Autodesk Inventor part; units mm, degrees
ref_plane "IDS_WORKPLANE{1}" through (-0.8, 0, 0) normal (1, 0, 0) x (0, 1, 0)
ref_plane "Work Plane2" through (3.5, 0, 0) normal (0, 0, -1) x (1, 0, 0)
ref_plane "YZ Plane" through (0, 0, 0) normal (1, 0, 0) x (0, 1, 0)
sketch "Sketch1" plane through (0, 0, 0) normal (0, 0, 1) x (1, 0, 0)
  line L0 (13, 0) -> (13, 1.75)
  line L1 (13, 1.75) -> (2.35, 1.75)
  line L2 (0.45, 3.65) -> (0, 3.65)
  line L3 (0, 3.65) -> (0, 0) construction
  arc A0 (0, 3.65) -> (-0.8, 0) centre (7.9266, 0) ccw
  line L4 (-3.7972, 0) -> (15.7995, 0)
  line L5 (0, -0.7387) -> (0, 4.432)
  line L6 (-0.8, 0) -> (-0.8, 3.65) construction
  line L7 (-0.8, 3.65) -> (0, 3.65) construction
  line L8 (0, 3.65) -> (0, 0)
  line L9 (-0.8, 0) -> (0, 0)
  line L10 (0, 0) -> (13, 0)
  line L11 (0.45, 3.65) -> (2.35, 1.75)
  dimension "d0" = 0.8
  dimension "d1" = 3.5
  dimension "d2" = 7.3
  dimension "d11" = 45
  dimension "d14" = 2.35
  dimension "d15" = 10.65
revolve "Body" add sketch "Sketch1" angle 360 about axis through (0, 0, 0) along (1, 0, 0)
ref_plane "IDS_WORKPLANE{1}" through (-0.8, 0, 0) normal (1, 0, 0) x (0, 1, 0)
sketch "Sketch2" plane through (-0.8, 0, 0) normal (1, 0, 0) x (0, 1, 0)
  line L0 (0, -5.11) -> (0, 5.11)
  line L1 (-5.11, 0) -> (5.11, 0)
  line L2 (0.5, -3.65) -> (-0.5, -3.65)
  line L3 (-0.5, -3.65) -> (-0.5, 3.65)
  line L4 (-0.5, 3.65) -> (0.5, 3.65)
  line L5 (0.5, 3.65) -> (0.5, -3.65)
  line L6 (0, 3.65) -> (0, -3.65) construction
  line L7 (-0.5, 0) -> (0.5, 0) construction
  circle A0 centre (0, 0) radius 3.65
  dimension "d8" = 1
extrude "Slot" cut sketch "Sketch2" along normal blind 1.4 contours A0 L3 L1 L0 | A0 L5 L2 | L2 L3 A0 | L0 L1 L5 A0 | L1 L3 A0 L0 | L0 A0 L5 L1 | A0 L3 L4 | L4 L5 A0
thread "Thread"
chamfer "Chamfer1" distance 1.75 distance2 3.2 1 edges at (13, -1.75, 0) measured on face at (13, -0.4366, 0.1076)
ref_plane "Work Plane2" through (3.5, 0, 0) normal (0, 0, -1) x (1, 0, 0)
equation "\"d0\" = KR"
equation "\"d1\" = NND"
equation "\"d2\" = KOD"
equation "\"d11\" = 0.5 * SEWI"
equation "\"d14\" = KOH"
equation "\"d15\" = GEL"
equation "\"d8\" = SBR"
equation "\"d9\" = STI"
equation "\"d3\" = GEL"
equation "\"d5\" = -0.5 * GD2 + 0.5 * NND"
equation "\"d6\" = SPTZ"
equation "\"NND\" = 3.5"
equation "\"GEL\" = 10.65"
equation "\"KOD\" = 7.3"
equation "\"KOH\" = 2.35"
equation "\"STI\" = 1.4"
equation "\"SBR\" = 1"
equation "\"KR\" = 0.8"
equation "\"SPTZ\" = 3.2"
equation "\"GD2\" = 0"
equation "\"SEWI\" = 90deg"
equation "\"d7\" = -KR"
equation "\"EPV\" = 4.1"
equation "\"THREADDIA\" = 3.5"
equation "\"TOA\" = 30deg"
equation "\"NLG\" = 13"
equation "\"PTC\" = 1.3"
equation "\"GD1\" = 2.64"
properties part number "ISO 1483 - ST3.5 x 13 - C" material "Steel"
Work out the finished part from the listing and answer in its coordinate system (mm). A direction names the side the tool comes from. Coordinates: 2 decimals unless noted, no trailing zeros. Write each loop counter-clockwise with the first axis right and the second up, starting at its lowest first coordinate (ties: lowest second). Pieces come first, ordered by that corner, then holes.
Q1. Which of the six approach directions +Z, -Z, +X, -X, +Y, -Y give full straight-line access (tool end or side, diameter ignored) to faces 5 (the face through (0, -0.5, 0)), 6 (the face through (6.023, 1.617, 0.67))?
Q2. A cutting plane is placed at B-B, the plane x = 7.5. Give the vertices of the cut face in (y, z).
Q3. Find the intervals of material crossed by line 1 (X direction, y = -3, z = -0.5); line 2 (X direction, y = -2.5, z = 1); line 3 (Y direction, x = 8.25, z = -0.75), in increasing order.
Q4. Each of these flat-tipped pins is pushed along its axis until it touches: pin 1 Ø1.5 at (x, z) = (7, 2) entering from +Y; pin 2 Ø1.5 at (y, z) = (-1, 0) entering from -X; pin 3 Ø4 at (x, z) = (4.5, -2.5) entering from -Y. Where does it stop, or does it pass through?
Q5. Determine the mould class of faces 1 (the face through (2.231, -0.405, 1.824)), 2 (the face through (0.6, 0, 0)), 3 (the face through (0.22, 3.65, 0.07)), 4 (the face through (0.22, -3.65, -0.07)) for opening direction Y: released by +Y, released by -Y, zero draft, split by the parting line, or undercut.
Q6. A cutting plane is placed at A-A, the plane x = 1.5. Give the vertices of the cut face in (y, z), then the cut area to 3 significant figures.
Findings below:
1. face 5: +Z, -Z, -X
1. face 6: +X
2. outline: circle Ø3.5 at (0, 0)
3. line 1: x = -0.25 to 1.06
3. line 2: x = -0.37 to 1.41
3. line 3: y = -1.58 to 1.58
4. pin 1: stops at y = 1.22
4. pin 2: stops at x = -0.79
4. pin 3: stops at y = -1.68
5. face 1: split by the parting line
5. face 2: undercut
5. face 3: released by +Y
5. face 4: released by -Y
6. outline: circle Ø5.2 at (0, 0)
6. area: 21.2 mm2
